Build history of the part. All positions in model axes, mm. A direction names the side the tool comes from. Round coordinates to 2 decimals unless told otherwise and drop trailing zeros. Loops run counter-clockwise (first coordinate to the right, second up) from the corner with the lowest first, then second, coordinate; pieces in that order, holes last.
from build123d import *

# Parameters (mm, degrees)
F0_R     = 2.101025
F0_R_2   = 1.5875
F0_R_3   = 5.584671
F1_DEPTH = 3.175


with BuildPart() as f1:
    # F0 (on Front) → F1 (new body, symmetric)
    with BuildSketch(Plane.XZ):
        Polygon((-46.817864, -12.7), (-46.817864, 0), (-46.817864, 10), (-53.349793, 10), (-53.349793, -2), (-68.587884, -2), (-68.587884, -10.7), (-53.349793, -10.7), (-53.349793, -22.7), (-46.817864, -22.7), align=None)
        with Locations((-54.907676, -6.436401)):
            Circle(F0_R, mode=Mode.SUBTRACT)
        Polygon((11.442136, 0), (1.442136, 0), (-46.817864, 0), (-46.817864, -12.7), (0, -12.7), (10, -12.7), (17.071068, -5.628932), align=None)
        with Locations((-8.515809, -6.064869)):
            Circle(F0_R_2, mode=Mode.SUBTRACT)
        with Locations((7.333491, -6.064869)):
            Circle(F0_R_3, mode=Mode.SUBTRACT)
    extrude(amount=F1_DEPTH, both=True)


solid = f1.part
(1) Probe line 1 (X direction, y = -1, z = -8); line 2 (X direction, y = -0.75, z = -13.5); line 3 (Z direction, x = -61.5, y = 3). List the from-to ranges inside material, lowest first.
Responses:
line 1: x = -68.59 to -56.31, -53.5 to 2.09, 12.57 to 14.7
line 2: x = -53.35 to -46.82
line 3: z = -10.7 to -2
(2) Pull direction X, two halves, no side cores. Call faces 4 (the face through (-17, 0, 0)), 5 (the face through (-68.588, 0, -6)), 6 (the face through (-52.904, 0.044, -5.805)): +X half, -X half, draft (parallel to the pull), parting line (faces both ways), or undercut.
Responses:
face 4: draft
face 5: -X half
face 6: undercut
(3) Which spindle directions (+Z, -Z, +X, -X, +Y, -Y) get a long thin tool onto all of the face, cutting with end or side? Do faces 1 (the face through (-53.35, 0, 4)), 2 (the face through (-53.35, 0, -17)), 3 (the face through (-46.818, 0, 5)). Say none if no direction does.
Responses:
face 1: +Z, -X, +Y, -Y
face 2: -Z, -X, +Y, -Y
face 3: +Z, +X, +Y, -Y
(4) Slice it at A-A on x = -46. List the corners of the cut face in (y, z) (3 decimals), plus the area to 3 significant figures.
Responses:
outline: (-3.175, -12.7) - (3.175, -12.7) - (3.175, 0) - (-3.175, 0) - close
area: 80.6 mm2
(5) Slice it at B-B on y = -2. List the corners of the cut face in (x, z) (1 decimal).
Responses:
outline: (-68.6, -10.7) - (-53.3, -10.7) - (-53.3, -22.7) - (-46.8, -22.7) - (-46.8, -12.7) - (10, -12.7) - (17.1, -5.6) - (11.4, 0) - (-46.8, 0) - (-46.8, 10) - (-53.3, 10) - (-53.3, -2) - (-68.6, -2) - close; hole circle Ø4.2 at (-54.9, -6.4); hole circle Ø3.2 at (-8.5, -6.1); hole circle Ø11.2 at (7.3, -6.1)
(6) Pin check, flat tips, straight feed: P1, Ø1, axis at x = 5, y = -1.5, coming from the +Z side; P2, Ø5, axis at x = -54.91, z = -6.44, coming from the -Y side (3 decimals); P3, Ø3, axis at x = -8, z = 2.5, coming from the -Y side; P4, Ø3, axis at y = 0, z = -15, coming from the -X side. Stop position of each tip, or through.
Responses:
P1: stops at z = 0
P2: stops at y = -3.175
P3: passes through
P4: stops at x = -53.35
(7) Slice it at C-C on z = -16. List the corners of the cut face in (x, y) (3 decimals), plus the area to 3 significant figures.
Responses:
outline: (-53.35, -3.175) - (-46.818, -3.175) - (-46.818, 3.175) - (-53.35, 3.175) - close
area: 41.5 mm2
